Autodesk Inventor part; units mm, degrees
ref_plane "YZ Plane" through (0, 0, 0) normal (1, 0, 0) x (0, 1, 0)
ref_plane "XZ Plane" through (0, 0, 0) normal (0, 1, 0) x (-1, 0, 0)
ref_plane "XY Plane" through (0, 0, 0) normal (0, 0, 1) x (1, 0, 0)
sketch "Sketch2" plane through (0, 0, 0) normal (0, 0, 1) x (1, 0, 0)
  circle A0 centre (0, 0) radius 11.5
  circle A1 centre (0, 0) radius 21.5
  dimension "d0" = 23
  dimension "d1" = 10
extrude "Extrusion1" add sketch "Sketch2" along normal blind 2
sketch "Sketch3" plane through (0, 0, 2) normal (0, 0, 1) x (1, 0, 0)
  circle A0 centre (0, 0) radius 21.5 construction
  circle A1 centre (0, 0) radius 11.5 construction
  circle A2 centre (0, 0) radius 16.5 construction
  point P0 (0, 16.5)
  point P1 (-14.2894, 8.25)
  point P2 (-14.2894, -8.25)
  point P3 (0, -16.5)
  point P4 (14.2894, -8.25)
  point P5 (14.2894, 8.25)
  dimension "d13" = 33
  dimension "d16" = 360
hole "Hole1" at (-14.2894, 8.25, 2) at (0, 16.5, 2) at (14.2894, 8.25, 2) at (14.2894, -8.25, 2) at (0, -16.5, 2) at (-14.2894, -8.25, 2) direction (0, 0, -1) diameter 4.5 end through all
properties part number "P025" material "Polytetrafluoroethylene"
Model file for the job. Use its own axes, mm. Give positions to 0.01 mm unless a question says otherwise; leave off trailing zeros. Loops run counter-clockwise (first coordinate to the right, second up) from the corner with the lowest first, then second, coordinate; pieces in that order, holes last. Notation, with made-up numbers: M -6,86 L 30,86 A27 cw 30,102 Z; hole C -37.5,-31 d10. An arc over 180 degrees is marked long. Use one line per item in the form item = value.
Item 1: Slice it at D-D on x = 9. List the corners of the cut face in (y, z), and give its area (3 significant figures).
Filled in:
outline = M -19.53,0 L -7.16,0 L -7.16,2 L -19.53,2 Z; M 7.16,0 L 19.53,0 L 19.53,2 L 7.16,2 Z
area = 49.5 mm^2
Item 2: Slice it at B-B on x = 0. List the corners of the cut face in (y, z).
Filled in:
outline = M -21.5,0 L -18.75,0 L -18.75,2 L -21.5,2 Z; M -14.25,0 L -11.5,0 L -11.5,2 L -14.25,2 Z; M 11.5,0 L 14.25,0 L 14.25,2 L 11.5,2 Z; M 18.75,0 L 21.5,0 L 21.5,2 L 18.75,2 Z
Item 3: Drill centre lines: L1, parallel to Y at x = 0, z = 1; L2, parallel to Y at x = -13.5, z = 1.4; L3, parallel to X at y = 8.25, z = 1.2. Where is each one in solid material? Low to high.
Filled in:
L1 = -21.5 to -18.75, -14.25 to -11.5, 11.5 to 14.25, 18.75 to 21.5
L2 = -16.73 to -10.36, -6.14 to 6.14, 10.36 to 16.73
L3 = -19.85 to -16.54, -12.04 to -8.01, 8.01 to 12.04, 16.54 to 19.85
Item 4: Flat gauge pin, fed straight in: pin 1 Ø1 at (x, z) = (5, 1) entering from +Y. Where does the tip first touch, or does it go through?
Filled in:
pin_1 = 21.02
Item 5: Slice it at A-A on y = 0. List the corners of the cut face in (x, z).
Filled in:
outline = M -21.5,0 L -11.5,0 L -11.5,2 L -21.5,2 Z; M 11.5,0 L 21.5,0 L 21.5,2 L 11.5,2 Z
Item 6: Slice it at C-C on z = 1.35. List the corners of the cut face in (x, y), and give its area (3 significant figures).
Filled in:
outline = C 0,0 d43; hole C -14.29,-8.25 d4.5; hole C -14.29,8.25 d4.5; hole C 0,0 d23; hole C 0,-16.5 d4.5; hole C 0,16.5 d4.5; hole C 14.29,-8.25 d4.5; hole C 14.29,8.25 d4.5
area = 941 mm^2
Item 7: Two-plate mould, pull along X, no slides. Class faces 1 (the flat face through (9, -9, 2)), 2 (the cylindrical face through (-0.676, -18.646, 0.986)), 3 (the cylindrical face through (-2.799, -21.317, 0.986)): released by +X, released by -X, zero draft, split by the parting line, or undercut.
Filled in:
face_1 = zero draft
face_2 = undercut
face_3 = split by the parting line
